Verification items for the finished model (mm, model axes). Give positions to 0.01 mm unless a question says otherwise; leave off trailing zeros. Order: outer loops, then holes, each group sorted by start corner. A loop starts at its lowest first (then second) coordinate and runs counter-clockwise, first axis right, second up. Notation, with made-up numbers: (43.25, -25.75) -> (74.25, -25.75) arc R26 ccw to (74.25, 11.25) -> close; hole circle Ø7 at (1, 78.5). An arc over 180 degrees is marked (long way). Write each question's results on one line, items separated by ' | '. Start each with the question number.
1. Depth check by flat-ended pin: pin 1 Ø5 at (y, z) = (17, -57) entering from -X; pin 2 Ø10 at (y, z) = (13, -40.5) entering from +X; pin 3 Ø1 at (x, y) = (88, 26.5) entering from +Z. Enter the tip coordinate at first touch or a pass-through.
2. Material ranges on L1, parallel to Y at x = 46, z = -51; L2, parallel to Z at x = 21, y = 15; L3, parallel to X at y = 14.75, z = -11, recorded low to high. Write a range as from..to.
3. Cross-section at C-C, the plane y = 2.75. Enter the section's corners in (x, z), then the cut area to 3 significant figures.
4. Cross-section at B-B, the plane x = 36. Enter the section's corners in (y, z), then the cut area to 3 significant figures.
5. Cross-section at A-A, the plane y = 18.5. State how many separate pieces and enclosed holes the cut face has, then the cut area to 3 significant figures.
6. Cross-section at D-D, the plane z = -11. Enter the section's corners in (x, y), then the cut area to 3 significant figures.
from build123d import *

# Parameters (mm, degrees)
BOSS_EXTRUDE2_DEPTH      = 20
CUT_EXTRUDE1_START       = -15
CUT_EXTRUDE1_DEPTH       = 15
SKETCH4_W                = 114
SKETCH4_H                = 74
CUT_EXTRUDE2_DEPTH       = 15
SKETCH5_R                = 2
CUT_EXTRUDE3_DEPTH       = 154.948043183
BOSS_EXTRUDE3_DEPTH      = 1
BOSS_EXTRUDE3_DEPTH_BACK = 6
SKETCH8_W                = 26
SKETCH8_H                = 6
CUT_EXTRUDE4_DEPTH       = 2
CUT_EXTRUDE4_DEPTH_BACK  = 35
SKETCH6_R                = 1
SKETCH10_R               = 2
BOSS_EXTRUDE4_DEPTH      = 15
SKETCH11_R               = 1.5
CUT_EXTRUDE5_DEPTH       = 15
SKETCH12_W               = 80
SKETCH12_H               = 5
BOSS_EXTRUDE5_DEPTH      = 120
FILLET1_R                = 5
BOSS_EXTRUDE6_DEPTH      = 5
SKETCH14_R               = 3
BOSS_EXTRUDE7_DEPTH      = 4
SKETCH15_R               = 2
CUT_EXTRUDE6_DEPTH       = 10
SKETCH16_W               = 12
SKETCH16_H               = 8
CUT_EXTRUDE7_DEPTH       = 1
SKETCH17_W               = 10
SKETCH17_H               = 6
CUT_EXTRUDE8_DEPTH       = 4


with BuildPart() as part:
    # Sketch2 → Boss-Extrude2 (new body)
    with BuildSketch(Plane(origin=(0, 0, 0), x_dir=(1, 0, 0), z_dir=(0, 1, 0))):
        Polygon((0, 80), (0, 50), (0, 30), (0, 0), (120, 0), (120, 30), (120, 50), (120, 80), align=None)
        with BuildLine():
            ThreePointArc((0, 30), (-10, 40), (0, 50))
            Line((0, 50), (0, 30))
        make_face()
        with BuildLine():
            ThreePointArc((120, 30), (130, 40), (120, 50))
            Line((120, 50), (120, 30))
        make_face()
    extrude(amount=BOSS_EXTRUDE2_DEPTH)

    # Sketch3 → Cut-Extrude1 (cut)
    with BuildSketch(Plane(origin=(0, 20, 0), x_dir=(1, 0, 0), z_dir=(0, 1, 0)).offset(CUT_EXTRUDE1_START)):
        with BuildLine():
            Line((0, 50), (0, 30))
            ThreePointArc((0, 30), (-10, 40), (0, 50))
        make_face()
        with BuildLine():
            Line((120, 50), (120, 30))
            ThreePointArc((120, 30), (130, 40), (120, 50))
        make_face()
    extrude(amount=CUT_EXTRUDE1_DEPTH, mode=Mode.SUBTRACT)

    # Sketch4 → Cut-Extrude2 (cut)
    with BuildSketch(Plane(origin=(0, 20, 0), x_dir=(1, 0, 0), z_dir=(0, 1, 0))):
        with Locations((60, 40)):
            Rectangle(SKETCH4_W, SKETCH4_H)
    extrude(amount=-CUT_EXTRUDE2_DEPTH, mode=Mode.SUBTRACT)

    # Sketch5 → Cut-Extrude3 (cut, through all)
    with BuildSketch(Plane.XZ):
        with Locations(Location((-5, -40, 0), (0, 0, 270))):
            Circle(SKETCH5_R)
        with Locations(Location((125, -40, 0), (0, 0, 270))):
            Circle(SKETCH5_R)
    extrude(amount=-CUT_EXTRUDE3_DEPTH, mode=Mode.SUBTRACT)

    # Sketch8 → Boss-Extrude3 (add, two sides: drawn at the far end of the back side and taken through both)
    with BuildSketch(Plane(origin=(120, 0, 0), x_dir=(0, 0, -1), z_dir=(1, 0, 0)).offset(-BOSS_EXTRUDE3_DEPTH_BACK)):
        with Locations((63, 13)):
            Rectangle(SKETCH8_W, SKETCH8_H)
    extrude(amount=BOSS_EXTRUDE3_DEPTH + BOSS_EXTRUDE3_DEPTH_BACK)

    # Sketch6 → Cut-Extrude4 (cut, two sides: drawn at the far end of the back side and taken through both)
    with BuildSketch(Plane(origin=(120, 0, 0), x_dir=(0, 0, -1), z_dir=(1, 0, 0)).offset(-CUT_EXTRUDE4_DEPTH_BACK)):
        with Locations(Location((73, 13, 0), (0, 0, 180))):
            Circle(SKETCH6_R)
        with Locations(Location((57, 13, 0), (0, 0, 180))):
            Circle(SKETCH6_R)
        with Locations(Location((53, 13, 0), (0, 0, 180))):
            Circle(SKETCH6_R)
        with Locations(Location((65, 13, 0), (0, 0, 180))):
            Circle(SKETCH6_R)
        with Locations(Location((61, 13, 0), (0, 0, 180))):
            Circle(SKETCH6_R)
        with Locations(Location((69, 13, 0), (0, 0, 180))):
            Circle(SKETCH6_R)
    extrude(amount=CUT_EXTRUDE4_DEPTH + CUT_EXTRUDE4_DEPTH_BACK, mode=Mode.SUBTRACT)

    # Sketch10 → Boss-Extrude4 (add)
    with BuildSketch(Plane(origin=(0, 5, 0), x_dir=(1, 0, 0), z_dir=(0, 1, 0))):
        with Locations(Location((12, 69.718295326, 0), (0, 0, 270))):
            Circle(SKETCH10_R)
        with Locations(Location((12, 11, 0), (0, 0, 270))):
            Circle(SKETCH10_R)
        with Locations(Location((103, 69, 0), (0, 0, 270))):
            Circle(SKETCH10_R)
        with Locations(Location((103, 11, 0), (0, 0, 270))):
            Circle(SKETCH10_R)
    extrude(amount=BOSS_EXTRUDE4_DEPTH)

    # Sketch11 → Cut-Extrude5 (cut)
    with BuildSketch(Plane(origin=(0, 20, 0), x_dir=(1, 0, 0), z_dir=(0, 1, 0))):
        with Locations(Location((12, 69.718295326, 0), (0, 0, 270))):
            Circle(SKETCH11_R)
        with Locations(Location((103, 69, 0), (0, 0, 270))):
            Circle(SKETCH11_R)
        with Locations(Location((12, 11, 0), (0, 0, 270))):
            Circle(SKETCH11_R)
        with Locations(Location((103, 11, 0), (0, 0, 270))):
            Circle(SKETCH11_R)
    extrude(amount=-CUT_EXTRUDE5_DEPTH, mode=Mode.SUBTRACT)

    # Sketch12 → Boss-Extrude5 (add)
    with BuildSketch(Plane.ZY):
        with Locations((-40, 22.5)):
            Rectangle(SKETCH12_W, SKETCH12_H)
    extrude(amount=-BOSS_EXTRUDE5_DEPTH)

    # Fillet1
    fillet1_edges = [part.edges().sort_by_distance(p)[0] for p in [
        (120, 25, -40),
        (60, 25, -80),
        (60, 25, 0),
        (0, 25, -40),
    ]]
    fillet(fillet1_edges, radius=FILLET1_R)

    # Sketch13 → Boss-Extrude6 (add)
    with BuildSketch(Plane(origin=(0, 25, 0), x_dir=(1, 0, 0), z_dir=(0, 1, 0))):
        Polygon((81.531027272, 58.115293075), (80.819981957, 55), (81.531027272, 51.884706925), (83.523331973, 49.386435849), (86.402295679, 48), (89.597704321, 48), (92.476668027, 49.386435849), (94.468972728, 51.884706925), (95.180018043, 55), (94.468972728, 58.115293075), (92.476668027, 60.613564151), (89.597704321, 62), (86.402295679, 62), (83.523331973, 60.613564151), align=None)
        Polygon((95.180018043, 25), (94.468972728, 28.115293075), (92.476668027, 30.613564151), (89.597704321, 32), (86.402295679, 32), (83.523331973, 30.613564151), (81.531027272, 28.115293075), (80.819981957, 25), (81.531027272, 21.884706925), (83.523331973, 19.386435849), (86.402295679, 18), (89.597704321, 18), (92.476668027, 19.386435849), (94.468972728, 21.884706925), align=None)
    extrude(amount=BOSS_EXTRUDE6_DEPTH)

    # Sketch14 → Boss-Extrude7 (add)
    with BuildSketch(Plane(origin=(0, 25, 0), x_dir=(1, 0, 0), z_dir=(0, 1, 0))):
        with Locations(Location((52, 25, 0), (0, 0, 270))):
            Circle(SKETCH14_R)
        with Locations(Location((65, 25, 0), (0, 0, 270))):
            Circle(SKETCH14_R)
    extrude(amount=BOSS_EXTRUDE7_DEPTH)

    # Sketch15 → Cut-Extrude6 (cut)
    with BuildSketch(Plane(origin=(0, 25, 0), x_dir=(1, 0, 0), z_dir=(0, 1, 0))):
        with Locations(Location((52, 55, 0), (0, 0, 270))):
            Circle(SKETCH15_R)
        with Locations(Location((65, 55, 0), (0, 0, 270))):
            Circle(SKETCH15_R)
    extrude(amount=-CUT_EXTRUDE6_DEPTH, mode=Mode.SUBTRACT)

    # Sketch16 → Cut-Extrude7 (cut)
    with BuildSketch(Plane.ZY):
        with Locations((-66, 10)):
            Rectangle(SKETCH16_W, SKETCH16_H)
    extrude(amount=-CUT_EXTRUDE7_DEPTH, mode=Mode.SUBTRACT)

    # Sketch17 → Cut-Extrude8 (cut)
    with BuildSketch(Plane.ZY.offset(-1)):
        with Locations((-66, 10)):
            Rectangle(SKETCH17_W, SKETCH17_H)
    extrude(amount=-CUT_EXTRUDE8_DEPTH, mode=Mode.SUBTRACT)


solid = part.part
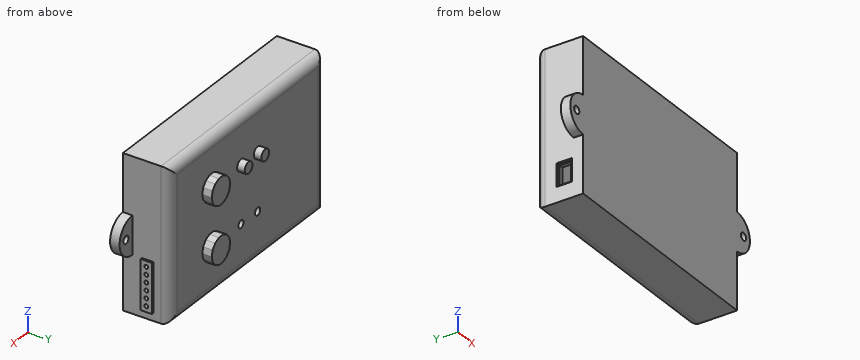
Results below:
1) pin 1: stops at x = 0 | pin 2: stops at x = 120 | pin 3: stops at z = -18
2) L1: y = 0..5, 20..25 | L2: z = -80..-77, -3..0 | L3: x = 0..3, 10..10.5, 13.5..14, 101..101.5, 104.5..105, 117..120
3) outline: (0, -80) -> (120, -80) -> (120, -50) arc R10 ccw to (120, -30) -> (120, 0) -> (0, 0) -> (0, -30) arc R10 ccw to (0, -50) -> close; hole circle Ø4 at (-5, -40); hole circle Ø4 at (125, -40) | area: 9,890 mm²
4) outline: (0, -80) -> (20, -80) arc R5 ccw to (25, -75) -> (25, -5) arc R5 ccw to (20, 0) -> (0, 0) -> close; hole (5, -77) -> (20, -77) -> (20, -3) -> (5, -3) -> close | area: 879 mm²
5) separate pieces: 5 | enclosed holes: 5 | area: 1,190 mm²
6) outline: (0, 0) -> (120, 0) -> (120, 20) arc R5 ccw to (115, 25) -> (5, 25) arc R5 ccw to (0, 20) -> close; hole (3, 5) -> (10, 5) -> (10, 20) -> (3, 20) -> close; hole (10.5, 5) -> (13.5, 5) -> (13.5, 20) -> (10.5, 20) -> close; hole (14, 5) -> (101, 5) -> (101, 20) -> (14, 20) -> close; hole (101.5, 5) -> (104.5, 5) -> (104.5, 20) -> (101.5, 20) -> close; hole (105, 5) -> (117, 5) -> (117, 20) -> (105, 20) -> close | area: 1,310 mm²
